CAD build for the part. Positions are in the model's coordinates, mm. Face numbers are marked on the shaded views. A direction names the side the tool comes from. Give positions to 0.01 mm unless a question says otherwise; leave off trailing zeros. Loops run counter-clockwise (first coordinate to the right, second up) from the corner with the lowest first, then second, coordinate; pieces in that order, holes last.
Item 1: Saw through at C-C on x = -12.5. Give the cut face in (y, z), plus the area to 3 significant figures.
Item 2: Which spindle directions (+Z, -Z, +X, -X, +Y, -Y) get a long thin tool onto all of the face, cutting with end or side? Do the marked faces 1, 2, 3 and 4. Say none if no direction does.
Item 3: Saw through at A-A on z = 0. Give the cut face in (x, y), plus the area to 4 significant figures.
Item 4: Saw through at B-B on y = -8.75. Give the cut face in (x, z).
Item 5: Saw through at D-D on z = 27. Give the cut face in (x, y), plus the area to 3 significant figures.
Item 6: Drop flat-ended pins along their axis: P1, Ø2, axis at y = -12, z = 41, coming from the +X side; P2, Ø3, axis at x = -13, y = -1.5, coming from the +Z side; P3, Ø2.5, axis at x = 0.5, z = 4, coming from the -Y side; P4, Ø10, axis at x = -12.5, z = 11, coming from the +Y side. Give the stop position or say it passes through.
Item 7: Probe probe 1 along X at (y, z) = (0.25, 0); probe 2 along X at (y, z) = (2.25, 0); probe 3 along Y at (x, z) = (-9.25, 73). List the from-to ranges inside material, lowest first.
from build123d import *

# Parameters (mm, degrees)
EXTRUDE_2_DEPTH     = 5
SKETCH_4_R          = 1.65
CUT_EXTRUDE_1_DEPTH = 5
EXTRUDE_3_DEPTH     = 5
CUT_EXTRUDE_START   = -4.5
SKETCH_7_R          = 3
CUT_EXTRUDE_2_DEPTH = 3
CUT_EXTRUDE_3_DEPTH = 7.5
EXTRUDE_4_DEPTH     = 5
FILLET_1_R          = 5
FILLET_2_R          = 5
EXTRUDE_5_DEPTH     = 15
EXTRUDE_6_DEPTH     = 5
CUT_EXTRUDE_START_2 = -5
CUT_EXTRUDE_4_DEPTH = 5


with BuildPart() as part:
    # 草图3 → 凸台-拉伸2 (new body)
    with BuildSketch(Plane(origin=(0, 0, 0), x_dir=(1, 0, 0), z_dir=(0, 1, 0))):
        with BuildLine():
            Line((-3, -3.354101966), (-3, -7.416198487))
            Line((-3, -7.416198487), (-3, -43.854101966))
            Line((-3, -43.854101966), (3, -43.854101966))
            Line((3, -43.854101966), (3, -10.583005244))
            Line((3, -10.583005244), (3, -7.416198487))
            Line((3, -7.416198487), (3, -3.354101966))
            ThreePointArc((3, -3.354101966), (0, 4.5), (-3, -3.354101966))
        make_face()
    extrude(amount=EXTRUDE_2_DEPTH)

    # 草图4 → 切除-拉伸1 (cut)
    with BuildSketch(Plane(origin=(0, 5, 0), x_dir=(1, 0, 0), z_dir=(0, 1, 0))):
        with Locations(Location((0, 0, 0), (0, 0, 270))):
            Circle(SKETCH_4_R)
    extrude(amount=-CUT_EXTRUDE_1_DEPTH, mode=Mode.SUBTRACT)

    # 草图6 → 凸台-拉伸3 (add)
    with BuildSketch(Plane(origin=(0, 5, 0), x_dir=(1, 0, 0), z_dir=(0, 1, 0))):
        with BuildLine():
            Line((3, -33.74604712), (-3, -33.74604712))
            ThreePointArc((-3, -33.74604712), (-16.46902092, -57.986607816), (0.722500961, -79.745993902))
            Line((0.722500961, -79.745993902), (1.949520222, -77.620734201))
            ThreePointArc((1.949520222, -77.620734201), (-10.543317179, -55.371702353), (3, -33.74604712))
        make_face()
    extrude(amount=-EXTRUDE_3_DEPTH)

    # 草图7 → 切除-拉伸2 (cut)
    with BuildSketch(Plane(origin=(0, 5, 0), x_dir=(1, 0, 0), z_dir=(0, 1, 0)).offset(CUT_EXTRUDE_START)):
        with Locations(Location((0, 0, 0), (0, 0, 270))):
            Circle(SKETCH_7_R)
    extrude(amount=-CUT_EXTRUDE_2_DEPTH, mode=Mode.SUBTRACT)

    # 草图8 → 切除-拉伸3 (cut)
    with BuildSketch(Plane(origin=(0, 5, 0), x_dir=(1, 0, 0), z_dir=(0, 1, 0))):
        with BuildLine():
            Line((-3, -38.067187498), (-3, -43.854101966))
            Line((-3, -43.854101966), (3, -43.854101966))
            Line((3, -43.854101966), (3, -33.74604712))
            ThreePointArc((3, -33.74604712), (-0.160637142, -35.683569047), (-3, -38.067187498))
        make_face()
    extrude(amount=-CUT_EXTRUDE_3_DEPTH, mode=Mode.SUBTRACT)

    # 草图9 → 凸台-拉伸4 (add)
    with BuildSketch(Plane(origin=(0, 5, 0), x_dir=(1, 0, 0), z_dir=(0, 1, 0))):
        with BuildLine():
            Line((-3, -18.550074543), (-14.614967684, -46.324924269))
            ThreePointArc((-14.614967684, -46.324924269), (-9.917875534, -39.010182445), (-3, -33.74604712))
            Line((-3, -33.74604712), (-3, -18.550074543))
        make_face()
    extrude(amount=-EXTRUDE_4_DEPTH)

    # 圆角1
    fillet_1_edges = [part.edges().sort_by_distance(p)[0] for p in [
        (3, 2.5, 33.74604712),
    ]]
    fillet(fillet_1_edges, radius=FILLET_1_R)

    # 圆角2
    # the kernel refuses this fillet: 5 mm, written as the material it takes off along each edge
    with BuildSketch(Plane(origin=(1.949520222, 14.371610933, 77.620734201), x_dir=(-0.8261015944022844, 0, -0.5635212114250925), z_dir=(0, -1, 0))) as fillet_2_piece_1:
        with BuildLine():
            CenterArc((4.123508811, -4.985927863), FILLET_2_R, 94.299664485, 55.185648669)
            Line((-0.183986354, -2.447131808), (-0.270136257, -2.396355887))
            ThreePointArc((-0.270136257, -2.396355887), (-0.191711734, -1.216068615), (-0.099718557, 0.007497289))
            Line((-0.099718557, 0.007497289), (0.007497289, 0.099718557))
            ThreePointArc((0.007497289, 0.099718557), (1.874322187, 0.029639314), (3.741147084, 0.099718557))
            Line((3.741147084, 0.099718557), (3.748644373, 0))
        make_face()
    extrude(amount=23.743221866, mode=Mode.SUBTRACT)

    # 草图10 → 凸台-拉伸5 (add)
    with BuildSketch(Plane.XZ):
        with BuildLine():
            Line((-3, 18.550074543), (3, 18.550074543))
            Line((3, 18.550074543), (3, 30.881988685))
            ThreePointArc((3, 30.881988685), (2.399314351, 33.25812699), (0.741586704, 35.063340422))
            ThreePointArc((0.741586704, 35.063340422), (-4.779586935, 39.993821756), (-8.614967684, 46.324924269))
            Line((-8.614967684, 46.324924269), (-14.614967684, 46.324924269))
            Line((-14.614967684, 46.324924269), (-3, 18.550074543))
        make_face()
    extrude(amount=EXTRUDE_5_DEPTH)

    # 草图11 → 凸台-拉伸6 (add)
    with BuildSketch(Plane.XZ.offset(15)):
        with BuildLine():
            Line((-14.614967684, 46.324924269), (-3, 18.550074543))
            Line((-3, 18.550074543), (3, 18.550074543))
            Line((3, 18.550074543), (3, 30.881988685))
            ThreePointArc((3, 30.881988685), (2.399314351, 33.25812699), (0.741586704, 35.063340422))
            ThreePointArc((0.741586704, 35.063340422), (-4.779586935, 39.993821756), (-8.614967684, 46.324924269))
            ThreePointArc((-8.614967684, 46.324924269), (-9.770106213, 62.167654699), (-1.147240872, 75.508293582))
            ThreePointArc((-1.147240872, 75.508293582), (0.307928877, 77.397579493), (0.722500961, 79.745993902))
            ThreePointArc((0.722500961, 79.745993902), (-14.272081884, 66.397409294), (-14.614967684, 46.324924269))
        make_face()
    extrude(amount=EXTRUDE_6_DEPTH)

    # 草图12 → 切除-拉伸4 (cut)
    with BuildSketch(Plane.XZ.offset(CUT_EXTRUDE_START_2)):
        with BuildLine():
            Line((-14.614967684, 46.324924269), (-8.614967684, 46.324924269))
            ThreePointArc((-8.614967684, 46.324924269), (-9.770106213, 62.167654699), (-1.147240872, 75.508293582))
            ThreePointArc((-1.147240872, 75.508293582), (0.307928877, 77.397579493), (0.722500961, 79.745993902))
            ThreePointArc((0.722500961, 79.745993902), (-14.272081884, 66.397409294), (-14.614967684, 46.324924269))
        make_face()
    extrude(amount=CUT_EXTRUDE_4_DEPTH, mode=Mode.SUBTRACT)


solid = part.part
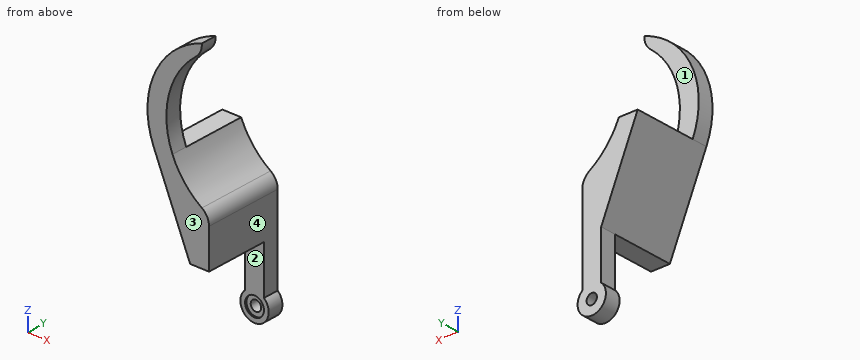
Results below:
1. outline: (-20, 41.27) - (5, 41.27) - (5, 46.32) - (-15, 46.32) - (-15, 69.61) - (-20, 69.61) - close
1. area: 243 mm2
2. face 1: +Z, +X, -X, +Y
2. face 2: -Z, +X, -X, -Y
2. face 3: +Z, -Z, +X, -X, -Y
2. face 4: +Z, +X, +Y, -Y
3. outline: (-4.5, 0) - (-3, 0) - (-3, 0.5) - (-1.65, 0.5) - (-1.65, 5) - (-4.5, 5) - close; (1.65, 0.5) - (3, 0.5) - (3, 0) - (4.5, 0) - (4.5, 5) - (1.65, 5) - close
3. area: 27.15 mm2
4. outline: (-14.61, 46.32) - (-3, 18.55) - (3, 18.55) - (3, 30.88) arc R5 ccw to (0.74, 35.06) arc R25 cw to (-8.61, 46.32) - close
5. outline: (-6.53, -20) - (3, -20) - (3, 5) - (-6.53, 5) - close
5. area: 238 mm2
6. P1: stops at x = -4.78
6. P2: stops at z = 46.32
6. P3: stops at y = 0
6. P4: passes through
7. probe 1: x = -4.5 to -3, 3 to 4.5
7. probe 2: x = -4.5 to -1.65, 1.65 to 4.5
7. probe 3: y = -20 to -15
